Can you work these out from the model? Positions are in its coordinate system, mm. Coordinates: 2 decimals unless noted, no trailing zeros. Loops run counter-clockwise (first coordinate to the right, second up) from the corner with the lowest first, then second, coordinate; pieces in that order, holes last. Notation, with made-up numbers: (-31, 55) -> (-13, 55) arc R11 cw to (-13, 67) -> close; hole circle Ø11 at (62, 86). An arc over 180 degrees is marked (long way). Use one line per item in the form item = value. Start each with the question number.
(1) Imagine slicing it at D-D (z = 1.75). List the corners of the cut face in (x, y) for me, plus the area to 3 significant figures.
(2) Imagine slicing it at C-C (y = -3.5). List the corners of the cut face in (x, z) for me.
(3) Imagine slicing it at A-A (x = -1.5). List the corners of the cut face in (y, z) for me, plus the area to 3 significant figures.
(4) I need wall thicknesses on line 1 (Y direction, x = 0, z = 2.85); line 2 (Y direction, x = 2.5, z = 1); line 3 (X direction, y = -0.5, z = 5). Which ranges of each line are inside material? Lowest first, please. Write a range as [from, to].
(5) I'm going to push flat-ended pins straight in: pin 1 (5 mm diameter, centred on x = 1, y = -1, fed in from +Z); pin 2 (1.5 mm diameter, centred on y = 2.5, z = 1, fed in from -X); pin 3 (3 mm diameter, centred on x = 6.5, z = 5.5, fed in from -Y). Where does each tip first touch, or does it pass through?
(6) Thinking about a two-plate mould opening in X: for faces 1 (the cylindrical face through (-3, 0, 3)), 2 (the cylindrical face through (-2.17, -9.76, 2.96)), 3 (the flat face through (2.1, 2.4, 0)), which applies, released by +X, released by -X, zero draft, split by the parting line, or undercut?
(7) Imagine slicing it at B-B (y = -0.25). List the corners of the cut face in (x, z) for me.
```python
from build123d import *

# Parameters (mm, degrees)
ESBO_O1_R                = 10
ESBO_O1_R_2              = 3
RESSALTO_EXTRUS_O1_DEPTH = 6
ESBO_O2_R                = 0.597777341
ESBO_O2_R_2              = 1.817872247
ESBO_O2_R_3              = 0.440898782
ESBO_O2_R_4              = 0.855469293
ESBO_O2_R_5              = 0.454468062
RESSALTO_EXTRUS_O2_DEPTH = 0.1


with BuildPart() as part:
    # Esboço1 → Ressalto-extrusão1 (new body)
    with BuildSketch(Plane.XY):
        Circle(ESBO_O1_R)
        Circle(ESBO_O1_R_2, mode=Mode.SUBTRACT)
    extrude(amount=RESSALTO_EXTRUS_O1_DEPTH)

    # Esboço2 → Ressalto-extrusão2 (add)
    with BuildSketch(Plane.XY.offset(6)):
        with Locations((-5.694217479, 4.731814525)):
            Circle(ESBO_O2_R)
        with Locations((0.668335385, 7.351689234)):
            Circle(ESBO_O2_R_2)
        with Locations((5.908084803, -4.999148679)):
            Circle(ESBO_O2_R_3)
        with Locations((-2.753541786, -2.967409109)):
            Circle(ESBO_O2_R_4)
        with Locations((-0.454468062, -7.939824373)):
            Circle(ESBO_O2_R_5)
    extrude(amount=RESSALTO_EXTRUS_O2_DEPTH)


solid = part.part
```
Worked out:
q1.outline = circle Ø20 at (0, 0); hole circle Ø6 at (0, 0)
q1.area = 286 mm2
q2.outline = (-9.37, 0) -> (9.37, 0) -> (9.37, 6) -> (-2.08, 6) -> (-2.08, 6.1) -> (-3.42, 6.1) -> (-3.42, 6) -> (-9.37, 6) -> close
q3.outline = (-9.89, 0) -> (-2.6, 0) -> (-2.6, 6) -> (-9.89, 6) -> close; (2.6, 0) -> (9.89, 0) -> (9.89, 6) -> (2.6, 6) -> close
q3.area = 87.5 mm2
q4.line_1 = [-10, -3], [3, 10]
q4.line_2 = [-9.68, -1.66], [1.66, 9.68]
q4.line_3 = [-9.99, -2.96], [2.96, 9.99]
q5.pin_1 = 6
q5.pin_2 = -9.85
q5.pin_3 = -8.66
q6.face_1 = undercut
q6.face_2 = split by the parting line
q6.face_3 = zero draft
q7.outline = (-10, 0) -> (-2.99, 0) -> (-2.99, 6) -> (-10, 6) -> close; (2.99, 0) -> (10, 0) -> (10, 6) -> (2.99, 6) -> close
